Verification items for the finished model (mm, model axes). A direction names the side the tool comes from. Give positions to 0.01 mm unless a question says otherwise; leave off trailing zeros. Loops run counter-clockwise (first coordinate to the right, second up) from the corner with the lowest first, then second, coordinate; pieces in that order, holes last. Notation, with made-up numbers: M 5,83.5 L 55,83.5 A26 ccw 55,102.5 Z; hole C 28,23 d1. An arc over 180 degrees is marked long. Answer in a Markdown table with one row per item.
```python
from build123d import *

# Parameters (mm, degrees)
CUT_EXTRUDE1_DEPTH = 1.6256


with BuildPart() as part:
    # Sketch5 → Revolve2 (revolve)
    with BuildSketch(Plane.XY):
        with BuildLine():
            Line((0, 1.080374022), (0, -12.7))
            Line((0, -12.7), (1.28016, -12.7))
            Line((1.28016, -12.7), (1.7526, -12.22756))
            Line((1.7526, -12.22756), (1.7526, -0.254))
            ThreePointArc((1.7526, -0.254), (1.826994878, -0.074394878), (2.0066, 0))
            Line((2.0066, 0), (2.8702, 0))
            Line((2.8702, 0), (2.8702, 3.1496))
            Line((2.8702, 3.1496), (2.5146, 3.5052))
            Line((2.5146, 3.5052), (1.3843, 3.5052))
            Line((1.3843, 3.5052), (1.3843, 1.8796))
            Line((1.3843, 1.8796), (0, 1.080374022))
        make_face()
    revolve(axis=Axis((0, 3.5052, 0), (0, 1, 0)))

    # Sketch3 → Cut-Extrude1 (cut)
    with BuildSketch(Plane(origin=(0, 3.5052, 0), x_dir=(1, 0, 0), z_dir=(0, 1, 0))):
        Polygon((-1.598451955, 0), (-0.799225978, -1.3843), (0.799225978, -1.3843), (1.598451955, 0), (0.799225978, 1.3843), (-0.799225978, 1.3843), align=None)
    extrude(amount=-CUT_EXTRUDE1_DEPTH, mode=Mode.SUBTRACT)


solid = part.part
```
Item 1: Go/stop test with flat-tipped pins: pin 1 (1.3 mm diameter, centred on x = -0.5, y = 2.5, fed in from +Z); pin 2 (1 mm diameter, centred on y = -1.5, z = 1.5, fed in from -X); pin 3 (1 mm diameter, centred on x = -2, y = -6, fed in from -Z). Record where each tip stops, or that it passes through.
Reported:
| item | result |
|---|---|
| pin 1 | stops at z = 2.87 |
| pin 2 | stops at x = -1.44 |
| pin 3 | stops at z = -0.91 |
Item 2: Tool access check on faces 5 (the flat face through (0, -12.7, 0)), 6 (the cylindrical face through (1.67, -6.16, -0.53)), 7 (the flat face through (1.193, 2.704, 0.702)). Record the directions out of +Z, -Z, +X, -X, +Y, -Y that give a thin tool (end or side, any length) a straight path to the whole face; none if there is none.
Reported:
| item | result |
|---|---|
| face 5 | +Z, -Z, +X, -X, -Y |
| face 6 | -Y |
| face 7 | +Y |
Item 3: Sectioned sample at B-B (y = -4.75). Record the cut outline in (x, z).
Reported:
| item | result |
|---|---|
| outline | C 0,0 d3.51 |
Item 4: Scan lines: L1, parallel to Y at x = -0.25, z = -2.2; L2, parallel to Z at x = 0.85, y = -3; L3, parallel to X at y = 2, z = 2.1. Record each from-to range of solid material in increasing order. Write a range as [from, to].
Reported:
| item | result |
|---|---|
| L1 | y = [0, 3.51] |
| L2 | z = [-1.53, 1.53] |
| L3 | x = [-1.96, 1.96] |
Item 5: Release check for a two-part mould opening along Z. For faces 1 (the flat face through (0, 3, -1.384)), 2 (the cylindrical face through (-2.278, 1.597, 1.746)), 3 (the flat face through (-1.193, 2.704, -0.702)), 4 (the flat face through (-1, 0, -2)) record: released by +Z, released by -Z, zero draft, split by the parting line, or undercut.
Reported:
| item | result |
|---|---|
| face 1 | undercut |
| face 2 | split by the parting line |
| face 3 | undercut |
| face 4 | zero draft |
Item 6: Sectioned sample at A-A (y = 0.5). Record the cut outline in (x, z), and give its area (3 significant figures).
Reported:
| item | result |
|---|---|
| outline | C 0,0 d5.74 |
| area | 25.9 mm^2 |
